Here's how the part is built. I have some questions about the finished solid (model axes, mm). A direction names the side the tool comes from. Coordinates: 2 decimals unless noted, no trailing zeros. Order: outer loops, then holes, each group sorted by start corner. A loop starts at its lowest first (then second) coordinate and runs counter-clockwise, first axis right, second up. Notation, with made-up numbers: (61, 84) - (103, 84) arc R9 ccw to (103, 95) - close; hole circle Ø3 at (47.5, 80). An arc over 180 degrees is marked (long way). Answer as CSV lines item,"result". Start each with the question number.
Q1. Suppose I cut it at D-D (y = 14.5). Please give me the cut outline in (x, z), then the cut area to 3 significant figures.
Q2. Suppose I cut it at C-C (z = -27.5). Please give me the cut outline in (x, y).
Q3. I need wall thicknesses on line 1 (Y direction, x = 11, z = -42); line 2 (Y direction, x = 37, z = -37). Which ranges of each line are inside material? Lowest first, please.
Q4. For faces 1 (the face through (12.7, 3, -51)), 2 (the face through (20, 3, 0)), 3 (the face through (37.509, 41.726, -42.706)), 4 (the face through (23, 41, -38.1)), 5 (the face through (23, 38.1, -41)), which set-ups out of +Z, -Z, +X, -X, +Y, -Y let a thin tool reach every point of the face, with its end or its side?
Q5. Suppose I cut it at A-A (y = 5.5). Please give me the cut outline in (x, z).
Q6. Thinking about a two-plate mould opening in X: for faces 6 (the face through (5, 34, 0)), 7 (the face through (6.025, 3.219, -49.336)), 8 (the face through (12.7, 3, 6)), 9 (the face through (34.29, 41, -3)), which applies, released by +X, released by -X, zero draft, split by the parting line, or undercut?
Q7. Suppose I cut it at B-B (z = 6.35). Please give me the cut outline in (x, y).
Q8. For pin 1 Ø2 at (y, z) = (7.5, -43) entering from +X; pin 2 Ø2 at (x, y) = (25, 6) entering from -Z; pin 3 Ø2.5 at (x, z) = (34.29, 6.35) entering from +Y; pin 4 Ø1.5 at (y, z) = (41.5, -2.5) entering from +X, each with a flat end and sliding along its axis, tell me the tip position at first contact or that it passes through.
from build123d import *

# Parameters (mm, degrees)
SKETCH1_W           = 40.64
SKETCH1_H           = 44.45
BOSS_EXTRUDE1_DEPTH = 44.45
SKETCH4_R           = 19.05
CUT_EXTRUDE3_DEPTH  = 41.64
SKETCH5_W           = 34.29
SKETCH5_H           = 38.1
CUT_EXTRUDE4_DEPTH  = 45.45
SKETCH6_W           = 6.35
SKETCH6_H           = 6.35
BOSS_EXTRUDE2_DEPTH = 34.29
SKETCH7_R           = 1.5
CUT_EXTRUDE5_DEPTH  = 6.35
SKETCH8_W           = 12.7
SKETCH8_H           = 6.35
BOSS_EXTRUDE3_DEPTH = 12.7
SKETCH10_R          = 1.5
CUT_EXTRUDE6_DEPTH  = 12.7


with BuildPart() as part:
    # Sketch1 → Boss-Extrude1 (new body)
    with BuildSketch(Plane(origin=(0, 0, 0), x_dir=(1, 0, 0), z_dir=(0, 1, 0))):
        with Locations((20.32, 22.225)):
            Rectangle(SKETCH1_W, SKETCH1_H)
    extrude(amount=BOSS_EXTRUDE1_DEPTH)

    # Sketch4 → Cut-Extrude3 (cut, through all)
    with BuildSketch(Plane.ZY):
        with Locations((-22.225, 22.225)):
            Circle(SKETCH4_R)
    extrude(amount=-CUT_EXTRUDE3_DEPTH, mode=Mode.SUBTRACT)

    # Sketch5 → Cut-Extrude4 (cut, through all)
    with BuildSketch(Plane(origin=(0, 0, -44.45), x_dir=(-1, 0, 0), z_dir=(0, 0, -1))):
        with Locations((-23.495, 25.4)):
            Rectangle(SKETCH5_W, SKETCH5_H)
    extrude(amount=-CUT_EXTRUDE4_DEPTH, mode=Mode.SUBTRACT)

    # Sketch6 → Boss-Extrude2 (add)
    with BuildSketch(Plane(origin=(6.35, 0, 0), x_dir=(0, 0, -1), z_dir=(1, 0, 0))):
        with Locations((3.175, 41.275)):
            Rectangle(SKETCH6_W, SKETCH6_H)
        with Locations((41.275, 41.275)):
            Rectangle(SKETCH6_W, SKETCH6_H)
    extrude(amount=BOSS_EXTRUDE2_DEPTH)

    # Sketch7 → Cut-Extrude5 (cut)
    with BuildSketch(Plane(origin=(40.64, 0, 0), x_dir=(0, 0, -1), z_dir=(1, 0, 0))):
        with Locations((3.175, 41.275)):
            Circle(SKETCH7_R)
        with Locations((41.275, 41.275)):
            Circle(SKETCH7_R)
        with Locations((41.275, 3.175)):
            Circle(SKETCH7_R)
        with Locations((3.175, 3.175)):
            Circle(SKETCH7_R)
    extrude(amount=-CUT_EXTRUDE5_DEPTH, mode=Mode.SUBTRACT)

    # Sketch8 → Boss-Extrude3 (add)
    with BuildSketch(Plane(origin=(0, 0, -44.45), x_dir=(-1, 0, 0), z_dir=(0, 0, -1))):
        with Locations((-34.29, 3.175)):
            Rectangle(SKETCH8_W, SKETCH8_H)
        with Locations((-6.35, 3.175)):
            Rectangle(SKETCH8_W, SKETCH8_H)
    boss_extrude3 = extrude(amount=BOSS_EXTRUDE3_DEPTH)

    # Sketch10 → Cut-Extrude6 (cut)
    with BuildSketch(Plane(origin=(0, 6.35, 0), x_dir=(1, 0, 0), z_dir=(0, 1, 0))):
        with Locations((6.35, 50.8)):
            Circle(SKETCH10_R)
        with Locations((34.29, 50.8)):
            Circle(SKETCH10_R)
    cut_extrude6 = extrude(amount=-CUT_EXTRUDE6_DEPTH, mode=Mode.SUBTRACT)

    # Mirror1: Boss-Extrude3, Cut-Extrude6 across plane
    add(boss_extrude3.mirror(Plane(origin=(0, 0, -22.225), x_dir=(1, 0, 0), z_dir=(0, 0, -1))))
    add(cut_extrude6.mirror(Plane(origin=(0, 0, -22.225), x_dir=(1, 0, 0), z_dir=(0, 0, -1))), mode=Mode.SUBTRACT)


solid = part.part
Here are the results:
1,outline,"(0, -44.45) - (6.35, -44.45) - (6.35, -39.64) - (0, -39.64) - close; (0, -4.81) - (6.35, -4.81) - (6.35, 0) - (0, 0) - close"
1,area,"61.1 mm²"
2,outline,"(0, 0) - (40.64, 0) - (40.64, 3.92) - (0, 3.92) - close; (0, 40.53) - (6.35, 40.53) - (6.35, 44.45) - (0, 44.45) - close"
3,line 1,"y = 0 to 6.35, 38.1 to 44.45"
3,line 2,"y = 0 to 6.35"
4,face 1,"-Z, +Y, -Y"
4,face 2,"+Z, +Y, -Y"
4,face 3,"+X"
4,face 4,"+X, +Y"
4,face 5,"+Z, -Z, +X"
5,outline,"(0, -57.15) - (12.7, -57.15) - (12.7, -44.45) - (27.94, -44.45) - (27.94, -57.15) - (40.64, -57.15) - (40.64, -31.35) - (0, -31.35) - close; (0, -13.1) - (40.64, -13.1) - (40.64, 12.7) - (27.94, 12.7) - (27.94, 0) - (12.7, 0) - (12.7, 12.7) - (0, 12.7) - close; hole circle Ø3 at (6.35, -50.8); hole circle Ø3 at (6.35, 6.35); hole circle Ø3 at (34.29, -50.8); hole circle Ø3 at (34.29, 6.35)"
6,face 6,"zero draft"
6,face 7,"undercut"
6,face 8,"undercut"
6,face 9,"released by +X"
7,outline,"(0, 0) - (4.85, 0) - (4.85, 6.35) - (0, 6.35) - close; (7.85, 0) - (12.7, 0) - (12.7, 6.35) - (7.85, 6.35) - close; (27.94, 0) - (32.79, 0) - (32.79, 6.35) - (27.94, 6.35) - close; (35.79, 0) - (40.64, 0) - (40.64, 6.35) - (35.79, 6.35) - close"
8,pin 1,"stops at x = 6.35"
8,pin 2,"stops at z = -44.45"
8,pin 3,"passes through"
8,pin 4,"stops at x = 34.29"
